Source: CAD feature listing. Evaluate the final solid. Frame: model axes, mm. A direction names the side the tool comes from. Give positions to 0.01 mm unless a question says otherwise; leave off trailing zeros. Write each loop counter-clockwise with the first axis right and the second up, starting at its lowest first coordinate (ties: lowest second). Pieces come first, ordered by that corner, then holes. Notation, with made-up numbers: (-20, 24.25) - (31, 24.25) arc R27 ccw to (31, 48.25) - close; hole circle Ø6 at (49.5, -27). An arc over 180 degrees is marked (long way). One line per question, with ' | ' between items. Start each with the question number.
(1) Pin query (flat end, axial travel): pin 1 (2.5 mm diameter, centred on y = -37.5, z = 4.5, fed in from -X); pin 2 (2.5 mm diameter, centred on y = -10, z = 4.5, fed in from +X); pin 3 (1.8 mm diameter, centred on y = -61.5, z = 4, fed in from -X). Return the tip coordinate at first contact, or that it passes through.
(2) Section D-D, the plane x = 10.5. Return loops of the section in (y, z), plus the area to 3 significant figures.
(3) Draft query along Y for faces 1 (the flat face through (5, -67.47, 4)), 2 (the cylindrical face through (17.056, 7.669, 3.863)), 3 (the flat face through (-51, -59.923, 4)). Return one class per face: +Y half, -Y half, draft (parallel to the pull), parting line (faces both ways), or undercut.
(4) Section C-C, the plane z = 3.81. Return loops of the section in (x, y), plus the area to 3 significant figures.
(5) Section B-B, the plane x = -42.5. Return loops of the section in (y, z), plus the area to 3 significant figures.
(6) Ray query, line 1 (X direction, y = -35.5, z = 5.75); line 2 (X direction, y = -45, z = 7); line 3 (Y direction, x = -37.5, z = 3). Return the intervals inside material, ascending. Write a range as [from, to].
(7) Access query for faces 4 (the flat face through (-39, -54.77, 4)), 5 (the cylindrical face through (-16.333, 8.005, 0.764)), 6 (the flat face through (-51, -63, 5.611)), 7 (the flat face through (-8.82, -14, 4)). Directions: +Z, -Z, +X, -X, +Y, -Y. A direction counts if a zero-diameter tool reaches every point of the face in a straight line with its end or side. Return the directions, or none.
(8) Section A-A, the plane y = -24.5. Return loops of the section in (x, z).
```python
from build123d import *

# Parameters (mm, degrees)
SKETCH1_R           = 1.27
BOSS_EXTRUDE1_DEPTH = 7.62
FILLET1_R           = 2.54
FILLET2_R           = 2.54
FILLET3_R           = 2.54
SKETCH4_R           = 2.667
BOSS_EXTRUDE2_DEPTH = 5.08
SKETCH5_W           = 3.683
SKETCH5_H           = 5.461
CUT_EXTRUDE2_DEPTH  = 8.89


with BuildPart() as part:
    # Sketch1 → Boss-Extrude1 (new body)
    with BuildSketch(Plane.XY):
        Polygon((-55.174879418, -67.47023925), (-55.174879418, -54.77023925), (-24.059879418, -54.77023925), (-24.059879418, 8.72976075), (-8.819879418, 8.72976075), (-8.819879418, -35.72023925), (16.580120582, -35.72023925), (16.580120582, 8.72976075), (31.820120582, 8.72976075), (31.820120582, -54.77023925), (62.935120582, -54.77023925), (62.935120582, -67.47023925), align=None)
        with Locations(Location((-42.474879418, -61.12023925, 0), (0, 0, 180))):
            Circle(SKETCH1_R, mode=Mode.SUBTRACT)
        with Locations(Location((50.235120582, -61.12023925, 0), (0, 0, 180))):
            Circle(SKETCH1_R, mode=Mode.SUBTRACT)
    extrude(amount=BOSS_EXTRUDE1_DEPTH)

    # Fillet1
    fillet1_edges = [part.edges().sort_by_distance(p)[0] for p in [
        (-16.439879418, 8.72976075, 0),
        (24.200120582, 8.72976075, 0),
        (24.200120582, 8.72976075, 7.62),
        (-24.059879418, 8.72976075, 3.81),
        (-8.819879418, 8.72976075, 3.81),
        (16.580120582, 8.72976075, 3.81),
        (31.820120582, 8.72976075, 3.81),
        (-16.439879418, 8.72976075, 7.62),
    ]]
    fillet(fillet1_edges, radius=FILLET1_R)

    # Fillet2
    fillet2_edges = [part.edges().sort_by_distance(p)[0] for p in [
        (3.880120582, -67.47023925, 0),
        (3.880120582, -67.47023925, 7.62),
    ]]
    fillet(fillet2_edges, radius=FILLET2_R)

    # Fillet3
    fillet3_edges = [part.edges().sort_by_distance(p)[0] for p in [
        (-55.174879418, -54.77023925, 3.81),
        (62.935120582, -54.77023925, 3.81),
    ]]
    fillet(fillet3_edges, radius=FILLET3_R)

    # Sketch4 → Boss-Extrude2 (add)
    with BuildSketch(Plane(origin=(62.935120582, 0, 0), x_dir=(0, 0, -1), z_dir=(1, 0, 0))):
        with Locations(Location((-3.81, -62.250449816, 0), (0, 0, 180))):
            Circle(SKETCH4_R)
    extrude(amount=BOSS_EXTRUDE2_DEPTH)

    # Sketch5 → Cut-Extrude2 (cut)
    with BuildSketch(Plane.ZY.offset(55.174879418)):
        with Locations((3.769019213, -62.653923663)):
            Rectangle(SKETCH5_W, SKETCH5_H)
    extrude(amount=-CUT_EXTRUDE2_DEPTH, mode=Mode.SUBTRACT)


solid = part.part
```
Check sheet entries:
1) pin 1: x = -24.06 | pin 2: x = 31.82 | pin 3: x = -46.28
2) outline: (-67.47, 2.54) arc R2.54 ccw to (-64.93, 0) - (-35.72, 0) - (-35.72, 7.62) - (-64.93, 7.62) arc R2.54 ccw to (-67.47, 5.08) - close | area: 239 mm²
3) face 1: -Y half | face 2: +Y half | face 3: undercut
4) outline: (-55.17, -67.47) - (62.94, -67.47) - (62.94, -64.92) - (68.02, -64.92) - (68.02, -59.58) - (62.94, -59.58) - (62.94, -57.31) arc R2.54 ccw to (60.4, -54.77) - (31.82, -54.77) - (31.82, 6.19) arc R2.54 ccw to (29.28, 8.73) - (19.12, 8.73) arc R2.54 ccw to (16.58, 6.19) - (16.58, -35.72) - (-8.82, -35.72) - (-8.82, 6.19) arc R2.54 ccw to (-11.36, 8.73) - (-21.52, 8.73) arc R2.54 ccw to (-24.06, 6.19) - (-24.06, -54.77) - (-52.63, -54.77) arc R2.54 ccw to (-55.17, -57.31) - (-55.17, -59.92) - (-46.28, -59.92) - (-46.28, -65.38) - (-55.17, -65.38) - close; hole circle Ø2.54 at (-42.47, -61.12); hole circle Ø2.54 at (50.24, -61.12) | area: 3,880 mm²
5) outline: (-67.47, 2.54) arc R2.54 ccw to (-64.93, 0) - (-62.39, 0) - (-62.39, 7.62) - (-64.93, 7.62) arc R2.54 ccw to (-67.47, 5.08) - close; (-59.85, 0) - (-54.77, 0) - (-54.77, 7.62) - (-59.85, 7.62) - close | area: 74.7 mm²
6) line 1: [-24.06, -8.82], [16.58, 31.82] | line 2: [-24.06, 31.82] | line 3: [-67.47, -54.77]
7) face 4: +Z, -Z, -X, +Y | face 5: -Z, +X, -X, +Y | face 6: -X | face 7: +Z, -Z, +Y
8) outline: (-24.06, 0) - (-8.82, 0) - (-8.82, 7.62) - (-24.06, 7.62) - close; (16.58, 0) - (31.82, 0) - (31.82, 7.62) - (16.58, 7.62) - close
